Geometry: final body of the model. Coordinates: model frame, mm. A direction names the side the tool comes from. Round coordinates to 2 decimals unless told otherwise and drop trailing zeros. Write each loop counter-clockwise with the first axis right and the second up, starting at its lowest first coordinate (ties: lowest second). Pieces come first, ordered by that corner, then holes. Notation, with made-up numbers: M -6.75,57 L 11.25,57 A22 cw 11.25,76 Z; hole C 50.5,86.25 d9. An arc over 180 degrees is marked long. Answer as CSV lines item,"result". Start each with the question number.
Q1. Ray query, probe 1 along Y at (x, z) = (-15, -95.5); probe 2 along Z at (x, y) = (-7.5, 5); probe 3 along Z at (x, y) = (-19, 9). Return the intervals inside material, ascending.
Q2. Section query D-D on y = 1.25. Output: boundary loops of the cut face in (x, z) (3 decimals).
Q3. Section query C-C on z = -93.75. Output: boundary loops of the cut face in (x, y).
Q4. Reachability of faces 4 (the cylindrical face through (-26.238, 6.549, -87.976)), 5 (the flat face through (-25, 10, -87)) from +Z, -Z, +X, -X, +Y, -Y: full face, straight path, thin tool, end or side. Return the list, or none.
Q5. Section query A-A on y = 6.25. Output: boundary loops of the cut face in (x, z) (3 decimals), and give its area (3 significant figures).
Q6. Mould query, pull axis X, two halves, no side actions, for faces 1 (the flat face through (-3.064, 5, -91)), 2 (the cylindrical face through (-27.5, 6.5, -94.9)), 3 (the flat face through (-28, 0, -92)). Classes: pulls with the +X half, pulls with the -X half, needs draft (parallel to the pull), parting line crosses it, or undercut.
Q7. First-contact query: pin 1 (6 mm diameter, centred on x = -44, y = 4.5, fed in from -Z); pin 2 (1.5 mm diameter, centred on x = -40, y = 6.5, fed in from +Z); pin 3 (3 mm diameter, centred on x = -15.5, y = 7, fed in from +Z). Flat tips, straight axial feed; report the tip coordinate or a pass-through.
Q8. Section query B-B on x = -23. Output: boundary loops of the cut face in (y, z), and give its area (3 significant figures).
```python
from build123d import *

# Parameters (mm, degrees)
BOSS_EXTRUDE1_DEPTH = 10
CUT_EXTRUDE1_DEPTH  = 7


with BuildPart() as part:
    # Sketch2 → Boss-Extrude1 (new body)
    with BuildSketch(Plane(origin=(0, 0, 0), x_dir=(1, 0, 0), z_dir=(0, 1, 0))):
        with BuildLine():
            Line((-51.50406107, 86.072206422), (-47.139527706, 78.778315244))
            Line((-47.139527706, 78.778315244), (-46.369315936, 77.491157977))
            ThreePointArc((-46.369315936, 77.491157977), (-25.527153744, 86.621922437), (-3.064253537, 90.252996489))
            Line((-3.064253537, 90.252996489), (-3.064253537, 91.753846651))
            Line((-3.064253537, 91.753846651), (-3.197123883, 100.254034452))
            ThreePointArc((-3.197123883, 100.254034452), (-28.254839769, 96.243218227), (-51.50406107, 86.072206422))
        make_face()
    extrude(amount=BOSS_EXTRUDE1_DEPTH)

    # Sketch4 → Cut-Extrude1 (cut)
    with BuildSketch(Plane(origin=(0, 10, 0), x_dir=(1, 0, 0), z_dir=(0, 1, 0))):
        with BuildLine():
            Line((-50.7338493, 84.785049155), (-47.139527706, 78.778315244))
            ThreePointArc((-47.139527706, 78.778315244), (-25.92674327, 88.067939731), (-3.064253537, 91.753846651))
            Line((-3.064253537, 91.753846651), (-3.173676414, 98.754016642))
            ThreePointArc((-3.173676414, 98.754016642), (-27.844000167, 94.800525735), (-50.7338493, 84.785049155))
        make_face()
    extrude(amount=-CUT_EXTRUDE1_DEPTH, mode=Mode.SUBTRACT)


solid = part.part
```
Entries:
1,probe 1,"y = 0 to 3"
1,probe 2,"z = -100.02 to -98.52, -91.5 to -89.99"
1,probe 3,"z = -98.49 to -96.96, -89.82 to -88.28"
2,outline,"M -51.504,-86.072 A100.305 ccw -3.197,-100.254 L -3.064,-91.754 L -3.064,-90.253 A90.305 cw -46.369,-77.491 Z"
3,outline,"M -35.67,0 L -3.1,0 L -3.1,3 L -31.2,3 L -31.2,10 L -35.67,10 Z"
4,face 4,"+Y"
4,face 5,"+Z, -Z, +X, -X, +Y"
5,outline,"M -51.504,-86.072 A100.305 ccw -3.197,-100.254 L -3.174,-98.754 A98.805 cw -50.734,-84.785 Z; M -47.14,-78.778 A91.805 ccw -3.064,-91.754 L -3.064,-90.253 A90.305 cw -46.369,-77.491 Z"
5,area,"145 mm^2"
6,face 1,"pulls with the +X half"
6,face 2,"undercut"
6,face 3,"needs draft"
7,pin 1,"stops at z = -91.54"
7,pin 2,"stops at z = -80.59"
7,pin 3,"stops at z = -88.69"
8,outline,"M 0,-97.63 L 10,-97.63 L 10,-96.09 L 3,-96.09 L 3,-88.88 L 10,-88.88 L 10,-87.33 L 0,-87.33 Z"
8,area,"52.6 mm^2"
